Check sheet for the drawn part. Datum: minimum x, y, z corner. Units: mm. Coordinates: 2 decimals unless noted, no trailing zeros. Order: outer loops, then holes, each group sorted by start corner. A loop starts at its lowest first (then second) coordinate and runs counter-clockwise, first axis right, second up.
1. Gauge pin test, flat ends, axial feed: pin 1 Ø1 at (y, z) = (86.5, 1) entering from -X (1 decimal); pin 2 Ø3 at (x, z) = (353, 4) entering from +Y (1 decimal); pin 3 Ø2 at (x, z) = (244, 4.5) entering from -Y. Record the tip position at first contact, or that the pin passes through.
2. Cross-section at C-C (y = 235). Enter the section's corners in (x, z).
3. Cross-section at D-D (y = 84.5). Enter the section's corners in (x, z).
4. Cross-section at B-B (z = 2). Enter the section's corners in (x, y) (1 decimal).
5. Thickness scan on line 1 (Y direction, x = 107.5, z = 3.5) (1 decimal); line 2 (Y direction, x = 206, z = 5.75) (1 decimal); line 3 (X direction, y = 270, z = 0.5) (1 decimal). Record the ranges inside material, lowest first.
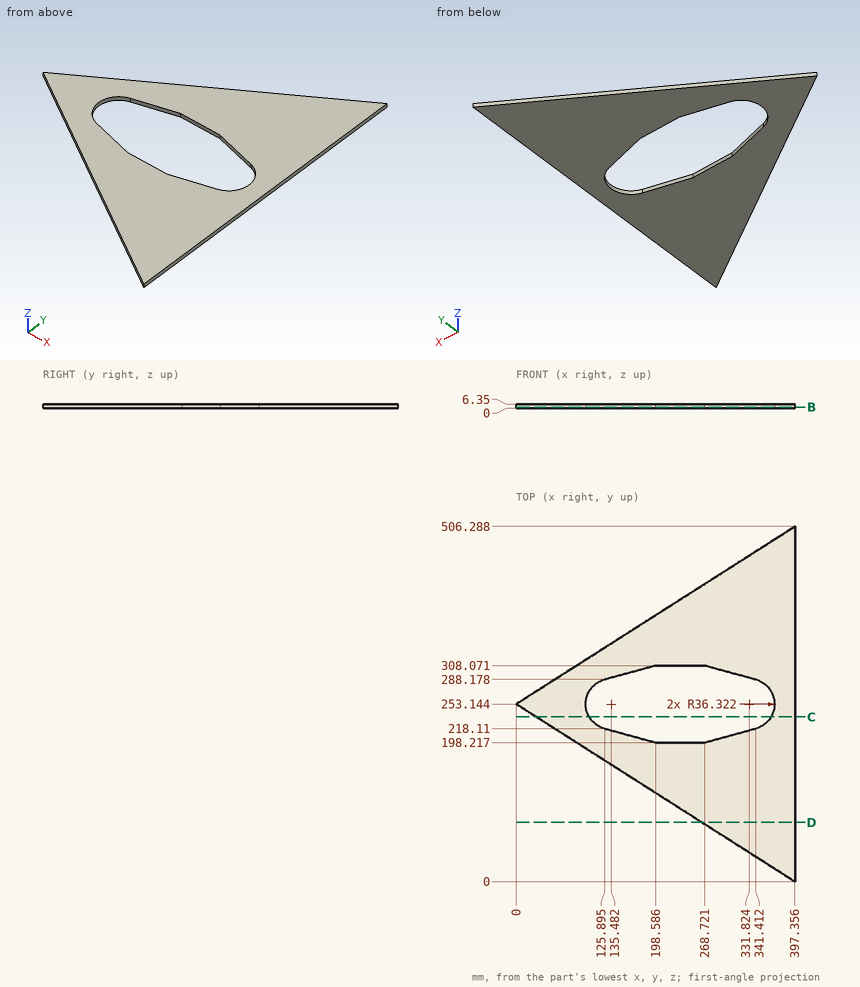
Data:
1. pin 1: stops at x = 260.8
1. pin 2: stops at y = 479
1. pin 3: stops at y = 97.06
2. outline: (28.48, 0) - (104.02, 0) - (104.02, 6.35) - (28.48, 6.35) - close; (363.29, 0) - (397.36, 0) - (397.36, 6.35) - (363.29, 6.35) - close
3. outline: (264.72, 0) - (397.36, 0) - (397.36, 6.35) - (264.72, 6.35) - close
4. outline: (0, 253.1) - (397.4, 0) - (397.4, 506.3) - close; hole (125.9, 218.1) - (198.6, 198.2) - (268.7, 198.2) - (341.4, 218.1) arc R36.3 ccw to (341.4, 288.2) - (268.7, 308.1) - (198.6, 308.1) - (125.9, 288.2) arc R36.3 ccw to start
5. line 1: y = 184.7 to 230, 276.3 to 321.6
5. line 2: y = 121.9 to 198.2, 308.1 to 384.4
5. line 3: x = 26.5 to 103.3, 364 to 397.4
